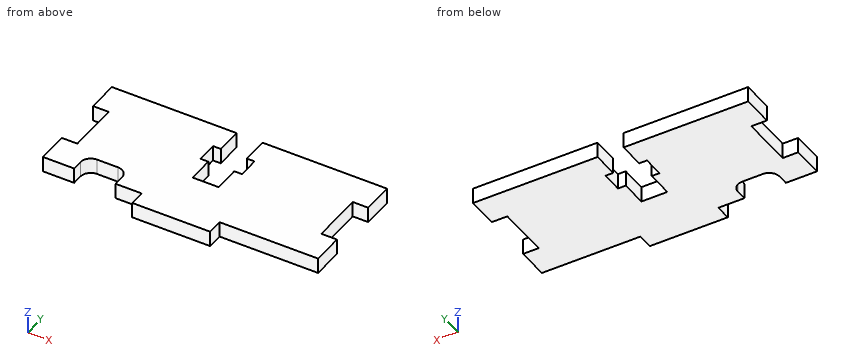
from build123d import *

# Parameters (mm, degrees)
BOSS_EXTRUDE1_DEPTH = 1.5
SKETCH2_W           = 3
SKETCH2_H           = 10
CUT_EXTRUDE1_DEPTH  = 56.865910894
SKETCH3_W           = 55
SKETCH3_H           = 25
CUT_EXTRUDE2_DEPTH  = 56.865910894
CUT_EXTRUDE3_DEPTH  = 56.865910894
CUT_EXTRUDE4_DEPTH  = 56.865910894


with BuildPart() as part:
    # Sketch1 → Boss-Extrude1 (new, symmetric)
    with BuildSketch(Plane.XY):
        Polygon((-20, -11), (20, -11), (20, -14), (35, -14), (35, -11), (54, -11), (54, 11), (-54, 11), (-54, -11), (-35, -11), (-35, -14), (-20, -14), align=None)
    extrude(amount=BOSS_EXTRUDE1_DEPTH, both=True)

    # Sketch2 → Cut-Extrude1 (cut, through all)
    with BuildSketch(Plane.XY.offset(1.5)):
        with Locations((2.5, 0)):
            Rectangle(SKETCH2_W, SKETCH2_H)
        with Locations((52.5, 0)):
            Rectangle(SKETCH2_W, SKETCH2_H)
    extrude(amount=-CUT_EXTRUDE1_DEPTH, mode=Mode.SUBTRACT)

    # Sketch3 → Cut-Extrude2 (cut, through all)
    with BuildSketch(Plane.XY.offset(1.5)):
        with Locations((-26.5, -1.5)):
            Rectangle(SKETCH3_W, SKETCH3_H)
    extrude(amount=-CUT_EXTRUDE2_DEPTH, mode=Mode.SUBTRACT)

    # Sketch4 → Cut-Extrude3 (cut, through all)
    with BuildSketch(Plane(origin=(0, 0, -1.5), x_dir=(-1, 0, 0), z_dir=(0, 0, -1))):
        with BuildLine():
            Line((-7, -11), (-7, -9))
            ThreePointArc((-7, -9), (-7.585786438, -7.585786438), (-9, -7))
            Line((-9, -7), (-13, -7))
            ThreePointArc((-13, -7), (-14.414213562, -7.585786438), (-15, -9))
            Line((-15, -9), (-15, -11))
            Line((-15, -11), (-7, -11))
        make_face()
    extrude(amount=-CUT_EXTRUDE3_DEPTH, mode=Mode.SUBTRACT)

    # Sketch5 → Cut-Extrude4 (cut, through all)
    with BuildSketch(Plane.XY.offset(1.5)):
        Polygon((25, 11), (25, 6), (23.5, 6), (23.5, 2), (25, 2), (25, -3), (30, -3), (30, 2), (31.5, 2), (31.5, 6), (30, 6), (30, 11), align=None)
    extrude(amount=-CUT_EXTRUDE4_DEPTH, mode=Mode.SUBTRACT)


solid = part.part
Build history of the part. All positions in model axes, mm. Round coordinates to 2 decimals unless told otherwise and drop trailing zeros. Write each loop counter-clockwise with the first axis right and the second up, starting at its lowest first coordinate (ties: lowest second). Pieces come first, ordered by that corner, then holes. Notation, with made-up numbers: (60.25, 55.25) -> (100.25, 55.25) arc R17 cw to (100.25, 73.25) -> close; hole circle Ø3 at (24.25, 28). An arc over 180 degrees is marked (long way). Write item = value, one per line.
(1) Band-saw the part on D-D (x = 6). Give the cut face in (y, z), then the cut area to 3 significant figures.
Answer:
outline = (-11, -1.5) -> (11, -1.5) -> (11, 1.5) -> (-11, 1.5) -> close
area = 66.0 mm2
(2) Flat gauge pins, fed straight in: pin 1 (1.5 mm diameter, centred on y = -0.5, z = -0.5, fed in from -X); pin 2 (1.5 mm diameter, centred on x = 43.5, z = -0.5, fed in from -Y); pin 3 (1.5 mm diameter, centred on y = -13, z = 0.5, fed in from +X). Where does each tip first touch, or does it go through?
Answer:
pin_1 = 4
pin_2 = -11
pin_3 = 35
(3) Band-saw the part on B-B (x = 30.5). Give the cut face in (y, z).
Answer:
outline = (-14, -1.5) -> (2, -1.5) -> (2, 1.5) -> (-14, 1.5) -> close; (6, -1.5) -> (11, -1.5) -> (11, 1.5) -> (6, 1.5) -> close
(4) Band-saw the part on A-A (y = 0.75). Give the cut face in (x, z).
Answer:
outline = (4, -1.5) -> (25, -1.5) -> (25, 1.5) -> (4, 1.5) -> close; (30, -1.5) -> (51, -1.5) -> (51, 1.5) -> (30, 1.5) -> close
(5) Probe L1, parallel to X at y = 2.25, z = -1.1; L2, parallel to X at y = 0.75, z = 0.4; L3, parallel to Y at x = 31, z = 1.2. List the from-to ranges inside material, lowest first.
Answer:
L1 = 4 to 23.5, 31.5 to 51
L2 = 4 to 25, 30 to 51
L3 = -14 to 2, 6 to 11
